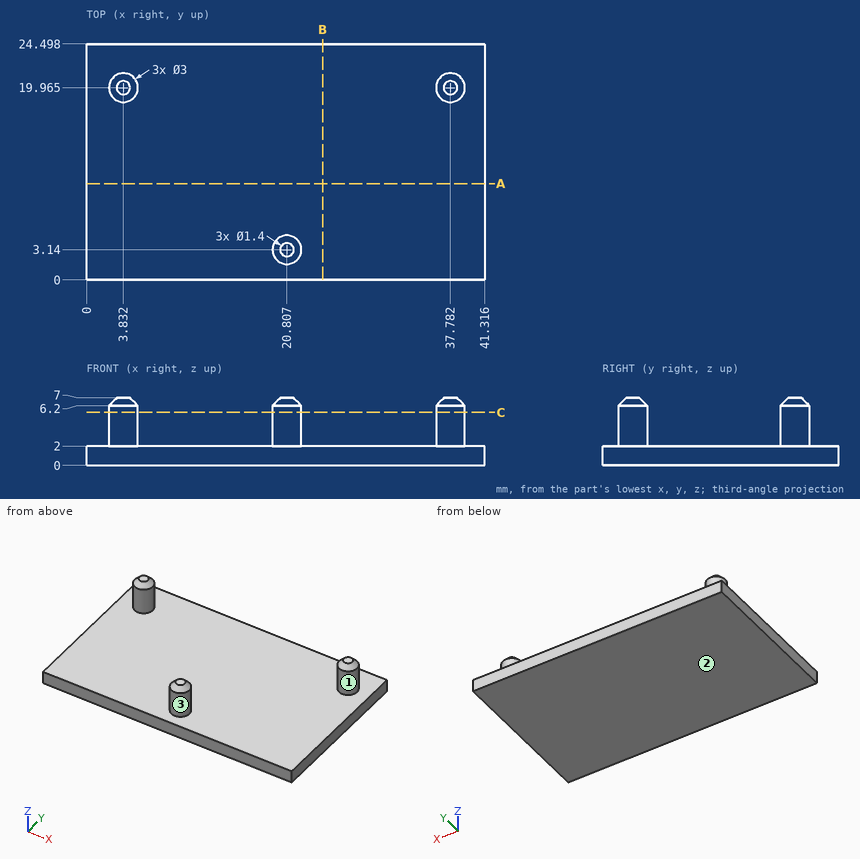
Geometry: see drawing. Coordinates: mm, zero at the bounding-box minimum. Coordinates: 2 decimals unless noted, no trailing zeros. Loops run counter-clockwise (first coordinate to the right, second up) from the corner with the lowest first, then second, coordinate; pieces in that order, holes last.
(1) Material intervals for probe 1 along Z at (x, y) = (9, 2.25); probe 2 along X at (y, z) = (20, 2.25), sorted ascending.
(2) First-contact query: pin 1 Ø5 at (x, y) = (27, 12) entering from -Z; pin 2 Ø1.5 at (x, y) = (8, 4.5) entering from +Z. Flat tips, straight axial feed; report the tip coordinate or a pass-through.
(3) Section B-B on x = 24.5. Return the cut outline in (y, z).
(4) Pull-direction query (X, two-part tool) for the marked faces 1, 2 and 3; classes: released by +X, released by -X, zero draft, split by the parting line, or undercut.
(5) Section C-C on z = 5.5. Return the cut outline in (x, y) (1 decimal), then the cut area to 3 significant figures.
(6) Section A-A on y = 10. Return the cut outline in (x, z).
Data:
1. probe 1: z = 0 to 2
1. probe 2: x = 2.33 to 5.33, 36.28 to 39.28
2. pin 1: stops at z = 0
2. pin 2: stops at z = 2
3. outline: (0, 0) - (24.5, 0) - (24.5, 2) - (0, 2) - close
4. face 1: undercut
4. face 2: zero draft
4. face 3: split by the parting line
5. outline: circle Ø3 at (3.8, 20); circle Ø3 at (20.8, 3.1); circle Ø3 at (37.8, 20)
5. area: 21.2 mm2
6. outline: (0, 0) - (41.32, 0) - (41.32, 2) - (0, 2) - close
